from build123d import *


with BuildPart() as part:
    # Sketch → Revolution (revolve)
    with BuildSketch(Plane.XY):
        with BuildLine():
            Line((0, -982.9308), (0, -1004.25873))
            ThreePointArc((0, -1004.25873), (8.885888, -1029.747625), (31.691892, -1044.188156))
            ThreePointArc((31.691892, -1044.188156), (125, -1054.92), (218.308108, -1044.188156))
            ThreePointArc((218.308108, -1044.188156), (241.114112, -1029.747625), (250, -1004.25873))
            Line((250, -982.9308), (250, -1004.25873))
            Line((235.857857, -968.788672), (250, -982.9308))
            ThreePointArc((235.857857, -968.788672), (125, -954.92), (14.142143, -968.788672))
            Line((14.142143, -968.788672), (0, -982.9308))
        make_face()
    revolve(axis=Axis((0, 0, 0), (1, 0, 0)))


solid = part.part
The model under review builds one solid part; all positions refer to its coordinate system, in mm. Coordinates: 2 decimals unless noted, no trailing zeros. Write each loop counter-clockwise with the first axis right and the second up, starting at its lowest first coordinate (ties: lowest second). Pieces come first, ordered by that corner, then holes. Notation, with made-up numbers: M 9.5,11.5 L 58.5,11.5 A12 ccw 58.5,20.5 Z; hole C 62,-25 d11. An arc over 180 degrees is marked long. Put each result on its own line as item: value.
1) Wall thickness on probe 1 along Z at (x, y) = (84, 493.5); probe 2 along Z at (x, y) = (18, 185); probe 3 along X at (y, z) = (744, -674.5): over which ranges is each line inside the solid? List them lowest first. Write a range as [from, to].
Computed:
probe 1: z = [-930.05, -819.7], [819.7, 930.05]
probe 2: z = [-1021.58, -949.98], [949.98, 1021.58]
probe 3: x = [0, 250]
2) Add section C-C on x = 155.5. Give the boundary of the cut face in (y, z).
Computed:
outline: C 0,0 d2107.57; hole C 0,0 d1911.91
3) Clearance check with flat-ended pins moving along their axes: pin 1 Ø1 at (x, y) = (175.5, -684.5) entering from -Z; pin 2 Ø12 at (x, z) = (34.5, 476) entering from -Y; pin 3 Ø8 at (x, z) = (56, 833) entering from +Y. State where each tip first meets the part, or that it passes through.
Computed:
pin 1: stops at z = -799.03
pin 2: stops at y = -933.5
pin 3: stops at y = 643.03
4) Draft analysis for pull direction Z (two halves, no side actions). For faces 1 (the flat face through (0, 739, 665)), 2 (the conical face through (13.26, 210.21, 946.61)), state which applies: released by +Z, released by -Z, zero draft, split by the parting line, or undercut.
Computed:
face 1: zero draft
face 2: undercut
5) Add section A-A on z = 0. Give the boundary of the cut face in (x, y).
Computed:
outline: M 0,-1004.26 A41 ccw 31.69,-1044.19 A411 ccw 218.31,-1044.19 A41 ccw 250,-1004.26 L 250,-982.93 L 235.86,-968.79 A450 ccw 14.14,-968.79 L 0,-982.93 Z; M 0,982.93 L 14.14,968.79 A450 ccw 235.86,968.79 L 250,982.93 L 250,1004.26 A41 ccw 218.31,1044.19 A411 ccw 31.69,1044.19 A41 ccw 0,1004.26 Z
